```python
from build123d import *

# Parameters (mm, degrees)
F1_DEPTH = 6.35
F2_R     = 3.17499
F3_R     = 1.6256
F4_DEPTH = 6.351
F5_R     = 1.6256
F6_DEPTH = 3.176


# Not quite as in the source:
# - a fillet or chamfer is up to 0.001 mm smaller than in the source, because OpenCascade refuses the exact size


with BuildPart() as f1:
    # F0 (on Top) → F1 (new body)
    with BuildSketch(Plane.XY):
        Polygon((0, 0), (0, -15.875), (6.35, -15.875), (6.35, -3.175), (28.575, -3.175), (28.575, 0), align=None)
    extrude(amount=F1_DEPTH)

    # F2 (radius 3.175 in the source; OpenCascade refuses exactly that, so slightly less here)
    f2_edges = [f1.edges().sort_by_distance(p)[0] for p in [
        (3.175, -15.875, 6.35),
        (3.175, -15.875, 0),
        (28.575, -1.5875, 6.35),
        (28.575, -1.5875, 0),
        (6.35, -3.175, 3.175),
    ]]
    fillet(f2_edges, radius=F2_R)

    # F3 (on face) → F4 (cut, through all)
    with BuildSketch(Plane.YZ.offset(6.35)):
        with Locations((-12.7, 3.175)):
            Circle(F3_R)
    extrude(amount=-F4_DEPTH, mode=Mode.SUBTRACT)

    # F5 (on face) → F6 (cut, through all)
    with BuildSketch(Plane.XZ.offset(3.175)):
        with Locations((25.4, 3.175)):
            Circle(F5_R)
    extrude(amount=-F6_DEPTH, mode=Mode.SUBTRACT)


solid = f1.part
```
Here's how the part is built. I have some questions about the finished solid (model axes, mm). A direction names the side the tool comes from. Give positions to 0.01 mm unless a question says otherwise; leave off trailing zeros. Order: outer loops, then holes, each group sorted by start corner. A loop starts at its lowest first (then second) coordinate and runs counter-clockwise, first axis right, second up. Notation, with made-up numbers: (64, 45) - (104, 45) arc R26 ccw to (104, 62) - close; hole circle Ø7 at (-14.5, -16). An arc over 180 degrees is marked (long way). Answer as a JSON object with one key per item and string values. Group by question number.
Item 1: If we section it at D-D on z = 5.25: Please give me the cut outline in (x, y) (3 decimals).
Item 2: For P1, Ø3, axis at x = 18.5, z = 2.5, coming from the -Y side (3 decimals); P2, Ø3, axis at y = -9.5, z = 3, coming from the +X side, each with a flat end and sliding along its axis, tell me the tip position at first contact or that it passes through.
Item 3: Please list where these lines run through material, in increasing order: probe 1 along Z at (x, y) = (5, -12.7); probe 2 along Y at (x, z) = (19.75, 5) (3 decimals); probe 3 along X at (y, z) = (-15, 2.25).
Item 4: If we section it at C-C on y = -9: Please give me the cut outline in (x, z).
Item 5: Which directions (+Z, -Z, +X, -X, +Y, -Y) give clear straight access to the entire face, cutting with the end or side of a thin tool? Please do faces 5 (the cylindrical face through (28, -2, 5)), 6 (the flat face through (19, -3.175, 3)).
Item 6: If we mould it in two halves opening along Z, with no side actions, what happens to faces 1 (the cylindrical face through (3.22, -11.2, 2.55)), 2 (the cylindrical face through (23.776, -1.61, 3.246)), 3 (the cylindrical face through (27.67, -1.565, 0.955)), 4 (the flat face through (14, 0, 3))? For each: pulls with the +Z half, pulls with the -Z half, needs draft (parallel to the pull), parting line crosses it, or undercut.
Item 7: If we section it at B-B on z = 2: Please give me the cut outline in (x, y) (3 decimals), and give its area (3 significant figures).
Result set:
{
 "1": {"outline": "(0, -15.103) - (6.35, -15.103) - (6.35, -6.35) arc R3.175 cw to (9.525, -3.175) - (27.803, -3.175) - (27.803, 0) - (0, 0) - close"},
 "2": {"P1": "y = -3.175", "P2": "x = 6.35"},
 "3": {"probe 1": "0 to 1.55, 4.8 to 6.35", "probe 2": "-3.175 to 0", "probe 3": "0 to 6.35"},
 "4": {"outline": "(0, 0) - (6.35, 0) - (6.35, 6.35) - (0, 6.35) - close"},
 "5": {"face 5": "+Z, +X, +Y, -Y", "face 6": "+Z, -Z, +X, -Y"},
 "6": {"face 1": "undercut", "face 2": "undercut", "face 3": "pulls with the -Z half", "face 4": "needs draft"},
 "7": {"outline": "(0, -15.65) - (6.35, -15.65) - (6.35, -13.823) - (0, -13.823) - close; (0, -11.577) - (6.35, -11.577) - (6.35, -6.35) arc R3.175 cw to (9.525, -3.175) - (24.277, -3.175) - (24.277, 0) - (0, 0) - close; (26.523, -3.175) - (28.35, -3.175) - (28.35, 0) - (26.523, 0) - close", "area": "150 mm²"}
}
